The listing builds one solid part. Answer for the finished solid, in the listing's coordinates (mm). A direction names the side the tool comes from. Coordinates: 2 decimals unless noted, no trailing zeros. Order: outer loops, then holes, each group sorted by start corner. A loop starts at its lowest first (then second) coordinate and runs counter-clockwise, first axis right, second up. Notation, with made-up numbers: (24, 52.5) -> (69, 52.5) arc R12 cw to (69, 71.5) -> close; hole circle Ø8 at (71.25, 40). An arc over 180 degrees is marked (long way). Write item = value, one per line. Start each with the question number.
```python
from build123d import *

# Parameters (mm, degrees)
F0_W     = 30
F0_H     = 10
F1_DEPTH = 10
F2_T     = -2.5


with BuildPart() as f1:
    # F0 (on Top) → F1 (new body)
    with BuildSketch(Plane.XY):
        Rectangle(F0_W, F0_H)
    extrude(amount=F1_DEPTH)

    # F2
    f2_openings = [f1.faces().sort_by_distance(p)[0] for p in [
        (0, 0, 10),
        (0, -5, 5),
    ]]
    offset(amount=F2_T, openings=f2_openings)


solid = f1.part
```
Item 1: Which of the six approach directions +Z, -Z, +X, -X, +Y, -Y give full straight-line access (tool end or side, diameter ignored) to faces 4 (the flat face through (0, 5, 5)), 5 (the flat face through (0, -1, 2.5))?
Item 2: Section A-A, the plane z = 7.25 is taken. Give the vertices of the cut face in (x, y).
Item 3: Consider probe 1 along X at (y, z) = (-3.75, 5); probe 2 along Y at (x, z) = (5.5, 7); probe 3 along Z at (x, y) = (-3, 1.75). Determine where each line is inside the solid, lowest interval first.
Item 4: For a pull along X with two mould halves and no side action, classify faces 1 (the flat face through (-12.5, -1, 6)), 2 (the flat face through (0, 3, 10)), 3 (the flat face through (15, 0, 5)) as pulls with the +X half, pulls with the -X half, needs draft (parallel to the pull), parting line crosses it, or undercut.
Item 5: Each of these flat-tipped pins is pushed along its axis until it touches: pin 1 (1 mm diameter, centred on x = 2, y = -2, fed in from -Z); pin 2 (6 mm diameter, centred on x = 4.5, y = -1.5, fed in from +Z). Where does it stop, or does it pass through?
Item 6: Section B-B, the plane y = -2.75 is taken. Give the vertices of the cut face in (x, z).
Item 7: Section C-C, the plane x = -5.75 is taken. Give the vertices of the cut face in (y, z), then the cut area to 4 significant figures.
A:
q1.face_4 = +Z, -Z, +X, -X, +Y
q1.face_5 = +Z, -Y
q2.outline = (-15, -5) -> (-12.5, -5) -> (-12.5, 2.5) -> (12.5, 2.5) -> (12.5, -5) -> (15, -5) -> (15, 5) -> (-15, 5) -> close
q3.probe_1 = -15 to -12.5, 12.5 to 15
q3.probe_2 = 2.5 to 5
q3.probe_3 = 0 to 2.5
q4.face_1 = undercut
q4.face_2 = needs draft
q4.face_3 = pulls with the +X half
q5.pin_1 = 0
q5.pin_2 = 2.5
q6.outline = (-15, 0) -> (15, 0) -> (15, 10) -> (12.5, 10) -> (12.5, 2.5) -> (-12.5, 2.5) -> (-12.5, 10) -> (-15, 10) -> close
q7.outline = (-5, 0) -> (5, 0) -> (5, 10) -> (2.5, 10) -> (2.5, 2.5) -> (-5, 2.5) -> close
q7.area = 43.75 mm^2
